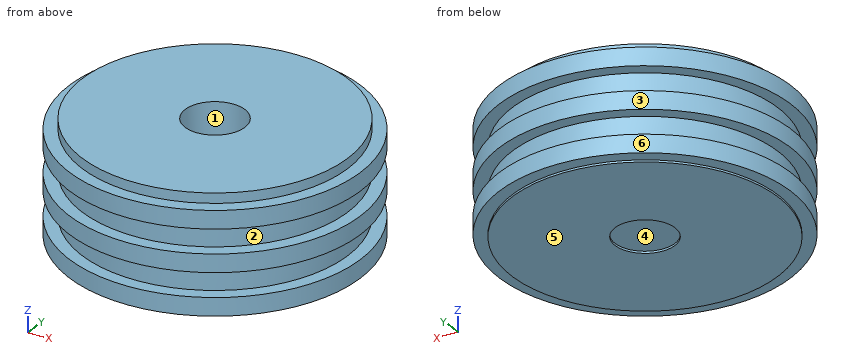
```python
from build123d import *

# Parameters (mm, degrees)
SKETCH1_R           = 66.675
SKETCH1_R_2         = 15
BOSS_EXTRUDE1_DEPTH = 57
SKETCH2_R           = 73.025
BOSS_EXTRUDE2_DEPTH = 9
SKETCH5_R           = 15
CUT_EXTRUDE1_DEPTH  = 116.625694593
LPATTERN3_COUNT     = 3
LPATTERN3_PITCH     = 21


with BuildPart() as part:
    # Sketch1 → Boss-Extrude1 (new body)
    with BuildSketch(Plane.XY):
        Circle(SKETCH1_R)
        Circle(SKETCH1_R_2, mode=Mode.SUBTRACT)
    extrude(amount=-BOSS_EXTRUDE1_DEPTH)

    # Sketch2 → Boss-Extrude2 (add)
    with BuildSketch(Plane.XY.offset(-5)):
        Circle(SKETCH2_R)
    boss_extrude2 = extrude(amount=-BOSS_EXTRUDE2_DEPTH)

    # Sketch5 → Cut-Extrude1 (cut, through all)
    with BuildSketch(Plane.XY.offset(-5)):
        Circle(SKETCH5_R)
    extrude(amount=-CUT_EXTRUDE1_DEPTH, mode=Mode.SUBTRACT)

    # LPattern3: Boss-Extrude2 ×3
    with Locations(*[(0, 0, -i * LPATTERN3_PITCH) for i in range(1, LPATTERN3_COUNT)]):
        add(boss_extrude2)


solid = part.part
```
Here's how the part is built. I have some questions about the finished solid (model axes, mm). Face numbers are marked on the shaded views. A direction names the side the tool comes from. Give positions to 0.01 mm unless a question says otherwise; leave off trailing zeros. Order: outer loops, then holes, each group sorted by start corner. A loop starts at its lowest first (then second) coordinate and runs counter-clockwise, first axis right, second up. Notation, with made-up numbers: (-40, 56.5) - (10, 56.5) arc R23 cw to (10, 88.5) - close; hole circle Ø8 at (22.5, 64). An arc over 180 degrees is marked (long way). Answer as a JSON object with one key per item and string values. Group by question number.
Item 1: Which directions (+Z, -Z, +X, -X, +Y, -Y) give clear straight access to the entire face, cutting with the end or side of a thin tool? Please do the marked faces 1, 2 and 3.
Item 2: For P1, Ø5, axis at y = 42.5, z = -24.5, coming from the -X side; P2, Ø4, axis at x = 51.5, z = -19.5, coming from the +Y side; P3, Ø6, axis at x = -54.5, y = 44, coming from the -Z side, each with a flat end and sliding along its axis, tell me the tip position at first contact or that it passes through.
Item 3: If we section it at B-B on y = 49: Please give me the cut outline in (x, z), and give its area (3 significant figures).
Item 4: If we section it at C-C on z = -32.5: Please give me the cut outline in (x, y) (3 decimals), and give its area (3 significant figures).
Item 5: Please list where these lines run through material, in increasing order: probe 1 along Z at (x, y) = (-29.5, 60); probe 2 along Y at (x, z) = (0, -39) (3 decimals); probe 3 along Y at (x, z) = (0, -8) (3 decimals).
Item 6: If we mould it in two halves opening along X, with no side actions, what happens to the marked faces 4, 5 and 6? For each: pulls with the +X half, pulls with the -X half, needs draft (parallel to the pull), parting line crosses it, or undercut.
Item 7: If we section it at A-A on x = 45.5: Please give me the cut outline in (y, z), and give its area (3 significant figures).
Result set:
{
 "1": {"face 1": "+Z", "face 2": "none", "face 3": "+Z, -Z"},
 "2": {"P1": "x = -60.77", "P2": "y = 44.67", "P3": "z = -56"},
 "3": {"outline": "(-54.14, -56) - (-45.22, -56) - (-45.22, -57) - (45.22, -57) - (45.22, -56) - (54.14, -56) - (54.14, -47) - (45.22, -47) - (45.22, -35) - (54.14, -35) - (54.14, -26) - (45.22, -26) - (45.22, -14) - (54.14, -14) - (54.14, -5) - (45.22, -5) - (45.22, 0) - (-45.22, 0) - (-45.22, -5) - (-54.14, -5) - (-54.14, -14) - (-45.22, -14) - (-45.22, -26) - (-54.14, -26) - (-54.14, -35) - (-45.22, -35) - (-45.22, -47) - (-54.14, -47) - close", "area": "5,640 mm²"},
 "4": {"outline": "circle Ø146.05 at (0, 0)", "area": "16,800 mm²"},
 "5": {"probe 1": "-56 to -47, -35 to -26, -14 to -5", "probe 2": "-66.675 to -15, 15 to 66.675", "probe 3": "-73.025 to -15, 15 to 73.025"},
 "6": {"face 4": "undercut", "face 5": "needs draft", "face 6": "parting line crosses it"},
 "7": {"outline": "(-57.12, -56) - (-48.74, -56) - (-48.74, -57) - (48.74, -57) - (48.74, -56) - (57.12, -56) - (57.12, -47) - (48.74, -47) - (48.74, -35) - (57.12, -35) - (57.12, -26) - (48.74, -26) - (48.74, -14) - (57.12, -14) - (57.12, -5) - (48.74, -5) - (48.74, 0) - (-48.74, 0) - (-48.74, -5) - (-57.12, -5) - (-57.12, -14) - (-48.74, -14) - (-48.74, -26) - (-57.12, -26) - (-57.12, -35) - (-48.74, -35) - (-48.74, -47) - (-57.12, -47) - close", "area": "6,010 mm²"}
}
